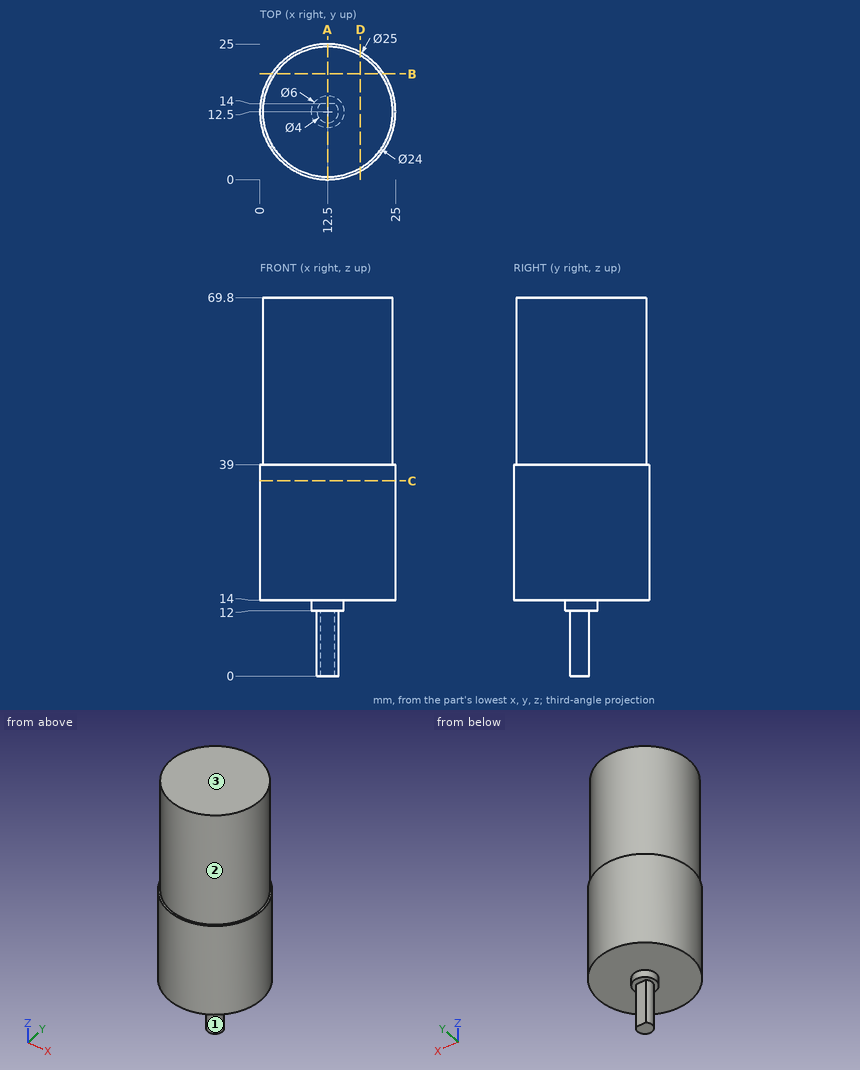
For this review, use the dimensioned drawing (mm, ordinates from the lowest corner) and the shaded views. A direction names the side the tool comes from. Coordinates: 2 decimals unless noted, no trailing zeros. Loops run counter-clockwise (first coordinate to the right, second up) from the corner with the lowest first, then second, coordinate; pieces in that order, holes last.
1. Add section B-B, the plane y = 19.5. Give the boundary of the cut face in (x, z).
2. For the marked faces 1, 2 and 3, list the 3-axis set-ups (+Z, -Z, +X, -X, +Y, -Y) from which the entire face can be reached by the end or side of a thin tool; tool diameter is ignored.
3. Insertion check: P1, Ø8, axis at x = 11.5, y = 21.5, coming from the -Z side; P2, Ø10, axis at y = 18, z = 16, coming from the -X side; P3, Ø2, axis at x = 10, z = 22.5, coming from the +Y side. Each pin has a flat end and moves straight along its axis. Give the tip position at first contact, or say it passes through.
4. Add section C-C, the plane z = 36. Give the boundary of the cut face in (x, y), then the cut area to 3 significant figures.
5. Add section A-A, the plane x = 12.5. Give the boundary of the cut face in (y, z).
6. For line 1 (Y direction, x = 16, z = 23); line 2 (Z direction, x = 16, y = 6.5); line 3 (Y direction, x = 7.25, z = 51.5), list the stretches that pass through material, from the lowest coordinate up.
7. Add section D-D, the plane x = 18.5. Give the boundary of the cut face in (y, z), then the cut area to 3 significant figures.
Result:
1. outline: (2.14, 14) - (22.86, 14) - (22.86, 39) - (22.25, 39) - (22.25, 69.8) - (2.75, 69.8) - (2.75, 39) - (2.14, 39) - close
2. face 1: -Z
2. face 2: +Z
2. face 3: +Z, +X, -X, +Y, -Y
3. P1: stops at z = 14
3. P2: stops at x = 0.01
3. P3: stops at y = 24.91
4. outline: circle Ø25 at (12.5, 12.5)
4. area: 491 mm2
5. outline: (0, 14) - (9.5, 14) - (9.5, 12) - (10.5, 12) - (10.5, 0) - (14, 0) - (14, 12) - (15.5, 12) - (15.5, 14) - (25, 14) - (25, 39) - (24.5, 39) - (24.5, 69.8) - (0.5, 69.8) - (0.5, 39) - (0, 39) - close
6. line 1: y = 0.5 to 24.5
6. line 2: z = 14 to 69.8
6. line 3: y = 1.71 to 23.29
7. outline: (1.53, 14) - (23.47, 14) - (23.47, 39) - (22.89, 39) - (22.89, 69.8) - (2.11, 69.8) - (2.11, 39) - (1.53, 39) - close
7. area: 1,190 mm2
